```python
from build123d import *

# Parameters (mm, degrees)
SKETCH2_R           = 12.7
BOSS_EXTRUDE1_DEPTH = 179.3
CHAMFER1_SIZE       = 1.5


with BuildPart() as part:
    # Sketch2 → Boss-Extrude1 (new, symmetric)
    with BuildSketch(Plane(origin=(0, 0, 0), x_dir=(0, 0, -1), z_dir=(1, 0, 0))):
        Circle(SKETCH2_R)
    extrude(amount=BOSS_EXTRUDE1_DEPTH, both=True)

    # Chamfer1
    chamfer1_edges = [part.edges().sort_by_distance(p)[0] for p in [
        (-179.3, 0, 12.7),
        (179.3, 0, 12.7),
    ]]
    chamfer(chamfer1_edges, length=CHAMFER1_SIZE)

    # Sketch5 → M10 Tapped Hole1 (revolve, cut)
    with BuildSketch(Plane(origin=(179.3, 0, 0), x_dir=(0, 0, -1), z_dir=(0, 1, 0))):
        Polygon((0, 0), (0, 27.053657631), (4.25, 24.5), (4.25, 20), (5, 20), (5, 1), (6, 0), align=None)
    m10_tapped_hole1 = revolve(axis=Axis((185.65, 0, 0), (-1, 0, 0)), mode=Mode.SUBTRACT)

    # Mirror1: M10 Tapped Hole1 across plane
    add(m10_tapped_hole1.mirror(Plane(origin=(0, 0, 0), x_dir=(0, 0, 1), z_dir=(1, 0, 0))), mode=Mode.SUBTRACT)


solid = part.part
```
For this review, take the finished solid that the model builds, in its own axes (mm). A direction names the side the tool comes from. Round coordinates to 2 decimals unless told otherwise and drop trailing zeros. Write each loop counter-clockwise with the first axis right and the second up, starting at its lowest first coordinate (ties: lowest second). Pieces come first, ordered by that corner, then holes. Notation, with made-up numbers: M -20,2.25 L 34,2.25 A28 cw 34,37.25 Z; hole C -17.75,-33 d11. An arc over 180 degrees is marked long. One line per item, written item: value. Start each with the question number.
(1) Wall thickness on line 1 (Z direction, x = -160.5, y = -0.25); line 2 (Y direction, x = 169.75, z = 0); line 3 (X direction, y = 3.5, z = -2.75): over which ranges is each line inside the solid? List them lowest first.
(2) We need section A-A (x = -106). Give the boundary of the cut face in (y, z).
(3) Insertion check: pin 1 (5 mm diameter, centred on y = -1.5, z = -1, fed in from -X); pin 2 (2 mm diameter, centred on x = 2, y = -10, fed in from +Z); pin 3 (10 mm diameter, centred on x = 32.5, y = -7, fed in from +Z). Each pin has a flat end and moves straight along its axis. Give the tip position at first contact, or say it passes through.
(4) The part is to be moulded in two halves that separate along Y. For faces 1 (the flat face through (179.3, -5, -5)), 2 (the cylindrical face through (2.49, -12.4, 2.75)), 3 (the cylindrical face through (168.93, 4.88, 1.08)), say which applies: released by +Y, released by -Y, zero draft, split by the parting line, or undercut.
(5) Machinability: for faces 4 (the flat face through (-179.3, -5, -5)), 5 (the flat face through (159.3, 4, -2)), 6 (the cylindrical face through (-168.93, 4.88, 1.08)), which of the approach directions +Z, -Z, +X, -X, +Y, -Y give a long, thin tool a straight path to every point of the face, cutting with its end or side? Answer none if there is none.
Result:
1. line 1: -12.7 to -4.99, 4.99 to 12.7
1. line 2: -12.7 to -5, 5 to 12.7
1. line 3: -159.3 to 159.3
2. outline: C 0,0 d25.4
3. pin 1: x = -159.3
3. pin 2: z = 8.96
3. pin 3: z = 12.54
4. face 1: zero draft
4. face 2: split by the parting line
4. face 3: undercut
5. face 4: +Z, -Z, -X, +Y, -Y
5. face 5: +X
5. face 6: -X
